Source: CAD feature listing. Evaluate the final solid. Frame: model axes, mm. Round coordinates to 2 decimals unless told otherwise and drop trailing zeros. Order: outer loops, then holes, each group sorted by start corner. A loop starts at its lowest first (then second) coordinate and runs counter-clockwise, first axis right, second up.
```python
from build123d import *

# Parameters (mm, degrees)
BOSS_EXTRUDE1_DEPTH = 6.35
SKETCH2_R           = 3.175
CUT_EXTRUDE1_DEPTH  = 700.833669971


with BuildPart() as part:
    # Sketch1 → Boss-Extrude1 (new body)
    with BuildSketch(Plane(origin=(0, 0, 0), x_dir=(1, 0, 0), z_dir=(0, 1, 0))):
        Polygon((122.428, 0), (122.428, -38.1), (483.997, -38.1), (483.997, 0), (606.425, 0), (606.425, 311.15), (483.997, 311.15), (483.997, 349.25), (122.428, 349.25), (122.428, 311.15), (0, 311.15), (0, 0), align=None)
    extrude(amount=BOSS_EXTRUDE1_DEPTH)

    # Sketch2 → Cut-Extrude1 (cut, through all)
    with BuildSketch(Plane(origin=(0, 6.35, 0), x_dir=(1, 0, 0), z_dir=(0, 1, 0))):
        with Locations(Location((498.983, 62.484, 0), (0, 0, 270))):
            Circle(SKETCH2_R)
    extrude(amount=-CUT_EXTRUDE1_DEPTH, mode=Mode.SUBTRACT)


solid = part.part
```
1. Section B-B on z = 8. Return loops of the section in (x, y).
2. First-contact query: pin 1 (8.5 mm diameter, centred on x = 498.983, z = -62.484, fed in from -Y); pin 2 (1.9 mm diameter, centred on y = 3, z = -322, fed in from -X); pin 3 (1.9 mm diameter, centred on x = 88, y = 3, fed in from -Z); pin 4 (1.9 mm diameter, centred on y = 2.5, z = -325.5, fed in from +X). Flat tips, straight axial feed; report the tip coordinate or a pass-through.
3. Line query: line 1 along Z through (x, y) = (511.5, 2.5); line 2 along X through (y, z) = (4.25, 5.5). Output: solid intervals per line, ascending.
4. Section A-A on y = 3.75. Return loops of the section in (x, z) (3 decimals).
5. Section C-C on x = 566.5. Return loops of the section in (y, z).
Result:
1. outline: (122.43, 0) - (484, 0) - (484, 6.35) - (122.43, 6.35) - close
2. pin 1: stops at y = 0
2. pin 2: stops at x = 122.43
2. pin 3: stops at z = -311.15
2. pin 4: stops at x = 484
3. line 1: z = -311.15 to 0
3. line 2: x = 122.43 to 484
4. outline: (0, -311.15) - (122.428, -311.15) - (122.428, -349.25) - (483.997, -349.25) - (483.997, -311.15) - (606.425, -311.15) - (606.425, 0) - (483.997, 0) - (483.997, 38.1) - (122.428, 38.1) - (122.428, 0) - (0, 0) - close; hole circle Ø6.35 at (498.983, -62.484)
5. outline: (0, -311.15) - (6.35, -311.15) - (6.35, 0) - (0, 0) - close
